CAD build for the part. Positions are in the model's coordinates, mm. Face numbers are marked on the shaded views. A direction names the side the tool comes from. Round coordinates to 2 decimals unless told otherwise and drop trailing zeros. Write each loop counter-clockwise with the first axis right and the second up, starting at its lowest first coordinate (ties: lowest second). Pieces come first, ordered by that corner, then holes. Notation, with made-up numbers: (-38.75, 29.25) -> (-17.75, 29.25) arc R17 ccw to (-17.75, 56.25) -> close; hole circle Ø8 at (74, -1.75). An arc over 180 degrees is marked (long way). Put each result on its own line as item: value. Start each with the question number.
1. Drill centre lines: line 1 (Z direction, x = 25, y = 3); line 2 (X direction, y = 1.8, z = -25); line 3 (X direction, y = 1.9, z = 0). Where is each one in solid material? Low to high. Write a range as from..to.
2. Saw through at B-B on x = -25. List the corners of the cut face in (y, z).
3. Saw through at C-C on x = 6.5. List the corners of the cut face in (y, z).
4. Saw through at A-A on z = -25. List the corners of the cut face in (x, y).
5. Flat gauge pins, fed straight in: P1, Ø9.5, axis at x = 25, z = -25, coming from the +Y side; P2, Ø5, axis at x = 2.5, y = 30, coming from the +Z side; P3, Ø8, axis at x = 25, z = 0, coming from the -Y side; P4, Ø14, axis at x = 3, z = 38.5, coming from the -Y side. Where does each tip first touch, or does it go through?
6. Saw through at D-D on y = 49.5. List the corners of the cut face in (x, z), and give its area (3 significant figures).
7. 3-axis set-ups, long thin cutter, end or side, ignore diameter. For the marked faces 1 and 2: which of +Z, -Z, +X, -X, +Y, -Y reach the whole face in a straight line?
from build123d import *

# Parameters (mm, degrees)
SKETCH_1_W      = 60
SKETCH_1_H      = 35
SKETCH_1_R      = 3
EXTRUDE_1_DEPTH = 5
SKETCH_2_R      = 3
EXTRUDE_2_DEPTH = 55
EXTRUDE_3_DEPTH = 14


with BuildPart() as part:
    # 스케치1 → 보스-돌출1 (new body)
    with BuildSketch(Plane(origin=(0, 0, 0), x_dir=(1, 0, 0), z_dir=(0, 1, 0))):
        with Locations((0, 12.5)):
            Rectangle(SKETCH_1_W, SKETCH_1_H)
        Circle(SKETCH_1_R, mode=Mode.SUBTRACT)
        with Locations((25, 0)):
            Circle(SKETCH_1_R, mode=Mode.SUBTRACT)
        with Locations((-25, 0)):
            Circle(SKETCH_1_R, mode=Mode.SUBTRACT)
        with Locations((25, 25)):
            Circle(SKETCH_1_R, mode=Mode.SUBTRACT)
        with Locations((0, 25)):
            Circle(SKETCH_1_R, mode=Mode.SUBTRACT)
        with Locations((-25, 25)):
            Circle(SKETCH_1_R, mode=Mode.SUBTRACT)
    extrude(amount=EXTRUDE_1_DEPTH)

    # 스케치2 → 보스-돌출2 (add)
    with BuildSketch(Plane.XZ):
        Circle(SKETCH_2_R)
    extrude(amount=-EXTRUDE_2_DEPTH)

    # 스케치3 → 보스-돌출3 (add)
    with BuildSketch(Plane(origin=(0, 55, 0), x_dir=(1, 0, 0), z_dir=(0, 1, 0))):
        with BuildLine():
            Line((8.75, 0), (8.75, -75))
            ThreePointArc((8.75, -75), (0, -83.75), (-8.75, -75))
            Line((-8.75, -75), (-8.75, 0))
            ThreePointArc((-8.75, 0), (0, 8.75), (8.75, 0))
        make_face()
    extrude(amount=-EXTRUDE_3_DEPTH)


solid = part.part
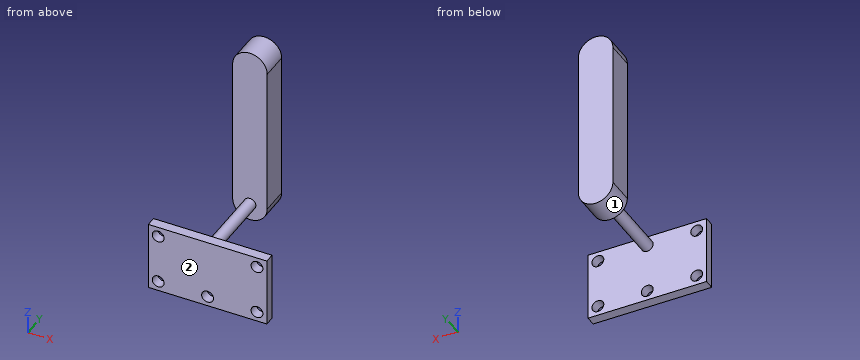
Return value:
1. line 1: z = -30..-28, -22..-3, 3..5
1. line 2: x = -30..-28, -22..-3, 3..22, 28..30
1. line 3: x = -30..-28, -22..22, 28..30
2. outline: (0, -30) -> (5, -30) -> (5, -28) -> (0, -28) -> close; (0, -22) -> (5, -22) -> (5, -3) -> (0, -3) -> close; (0, 3) -> (5, 3) -> (5, 5) -> (0, 5) -> close
3. outline: (0, -30) -> (5, -30) -> (5, 5) -> (0, 5) -> close; (41, -5.86) -> (55, -5.86) -> (55, 80.86) -> (41, 80.86) -> close
4. outline: (-30, 0) -> (-28, 0) -> (-28, 5) -> (-30, 5) -> close; (-22, 0) -> (-3, 0) -> (-3, 5) -> (-22, 5) -> close; (3, 0) -> (22, 0) -> (22, 5) -> (3, 5) -> close; (28, 0) -> (30, 0) -> (30, 5) -> (28, 5) -> close
5. P1: stops at y = 5
5. P2: stops at z = 3
5. P3: stops at y = 0
5. P4: stops at y = 41
6. outline: (-8.75, 0) arc R8.75 ccw to (8.75, 0) -> (8.75, 75) arc R8.75 ccw to (-8.75, 75) -> close
6. area: 1,550 mm^2
7. face 1: -Z, +Y
7. face 2: +Z, -Z, +X, -X, -Y
